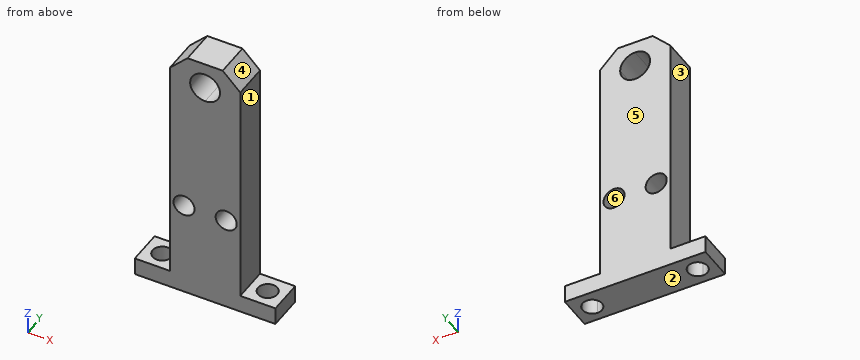
from build123d import *

# Parameters (mm, degrees)
F0_R     = 3
F1_DEPTH = 5
F2_SIZE  = 5
F4_DEPTH = 5


with BuildPart() as f1:
    # F0 (on Front) → F1 (new body, symmetric)
    with BuildSketch(Plane.XZ):
        Polygon((0, 37.5), (-10, 37.5), (-10, -37.5), (10, -37.5), (10, 37.5), align=None)
        with Locations((-6, -10)):
            Circle(F0_R, mode=Mode.SUBTRACT)
        with BuildLine():
            ThreePointArc((9, -10), (6, -13), (3, -10))
            ThreePointArc((3, -10), (6, -7), (9, -10))
        make_face(mode=Mode.SUBTRACT)
        with BuildLine():
            ThreePointArc((0, 25.75), (-4.25, 30), (0, 34.25))
            ThreePointArc((0, 34.25), (3.005204, 33.005204), (4.25, 30))
            ThreePointArc((4.25, 30), (3.005204, 26.994796), (0, 25.75))
        make_face(mode=Mode.SUBTRACT)
    extrude(amount=F1_DEPTH, both=True)

    # F2
    f2_edges = [f1.edges().sort_by_distance(p)[0] for p in [
        (-10, 0, 37.5),
        (10, 0, 37.5),
    ]]
    chamfer(f2_edges, length=F2_SIZE)

    # F3 (on face) → F4 (join)
    with BuildSketch(Plane(origin=(0, 0, -37.5), x_dir=(1, 0, 0), z_dir=(0, 0, -1))):
        Polygon((-10, -5), (-10, 5), (-15, 5), (-20, 5), (-20, -5), align=None)
        with BuildLine():
            ThreePointArc((-12.25, 0), (-16.944544, -1.944544), (-15, 2.75))
            ThreePointArc((-15, 2.75), (-13.055456, 1.944544), (-12.25, 0))
        make_face(mode=Mode.SUBTRACT)
        Polygon((15, 5), (10, 5), (10, -5), (20, -5), (20, 5), align=None)
        with BuildLine():
            ThreePointArc((17.75, 0), (13.055456, -1.944544), (15, 2.75))
            ThreePointArc((15, 2.75), (16.944544, 1.944544), (17.75, 0))
        make_face(mode=Mode.SUBTRACT)
    extrude(amount=-F4_DEPTH)


solid = f1.part
Build history of the part. All positions in model axes, mm. Face numbers are marked on the shaded views. A direction names the side the tool comes from. Round coordinates to 2 decimals unless told otherwise and drop trailing zeros. Order: outer loops, then holes, each group sorted by start corner. A loop starts at its lowest first (then second) coordinate and runs counter-clockwise, first axis right, second up. Notation, with made-up numbers: M -40,53.25 L -29,53.25 A10 cw -29,62.25 Z; hole C -38,-28.5 d2. An arc over 180 degrees is marked long. Use CSV: the item, a comma, the result in double quotes. Start each with the question number.
(1) Tool access for the marked faces 1, 2 and 3: list every direction of +Z, -Z, +X, -X, +Y, -Y with a clear straight run to the whole face (end or side of a thin tool).
(2) Cut at C-C on z = -10. List the corners of the cut face in (x, y).
(3) Cut at B-B on y = 3.75. List the corners of the cut face in (x, z).
(4) Flat gauge pins, fed straight in: P1, Ø6, axis at y = 4, z = 5.5, coming from the +X side; P2, Ø6, axis at y = -0.5, z = -22.5, coming from the -X side; P3, Ø3, axis at x = 16, y = 0, coming from the +Z side. Where does each tip first touch, or does it go through?
(5) Cut at D-D on z = -25.5. List the corners of the cut face in (x, y).
(6) Cut at A-A on x = 6. List the corners of the cut face in (y, z).
(7) Drill centre lines: probe 1 along X at (y, z) = (0, -33.9); probe 2 along Z at (x, y) = (-6.5, -3); probe 3 along Y at (x, z) = (-15, -34.3). Where is each one in solid material? Low to high.
(8) Mould opens along Z. For the marked faces 4, 5 and 6 say: +Z half, -Z half, draft (parallel to the pull), parting line (faces both ways), or undercut.
Findings:
1,face 1,"+Z, +X, +Y, -Y"
1,face 2,"-Z, +X, -X, +Y, -Y"
1,face 3,"+Z, -X, +Y, -Y"
2,outline,"M -10,-5 L -9,-5 L -9,5 L -10,5 Z; M -3,-5 L 3,-5 L 3,5 L -3,5 Z; M 9,-5 L 10,-5 L 10,5 L 9,5 Z"
3,outline,"M -20,-37.5 L 20,-37.5 L 20,-32.5 L 10,-32.5 L 10,32.5 L 5,37.5 L -5,37.5 L -10,32.5 L -10,-32.5 L -20,-32.5 Z; hole C -6,-10 d6; hole C 0,30 d8.5; hole C 6,-10 d6"
4,P1,"stops at x = 10"
4,P2,"stops at x = -10"
4,P3,"passes through"
5,outline,"M -10,-5 L 10,-5 L 10,5 L -10,5 Z"
6,outline,"M -5,-37.5 L 5,-37.5 L 5,-13 L -5,-13 Z; M -5,-7 L 5,-7 L 5,36.5 L -5,36.5 Z"
7,probe 1,"x = -20 to -17.75, -12.25 to 12.25, 17.75 to 20"
7,probe 2,"z = -37.5 to -12.96, -7.04 to 36"
7,probe 3,"y = -5 to -2.75, 2.75 to 5"
8,face 4,"+Z half"
8,face 5,"draft"
8,face 6,"undercut"
